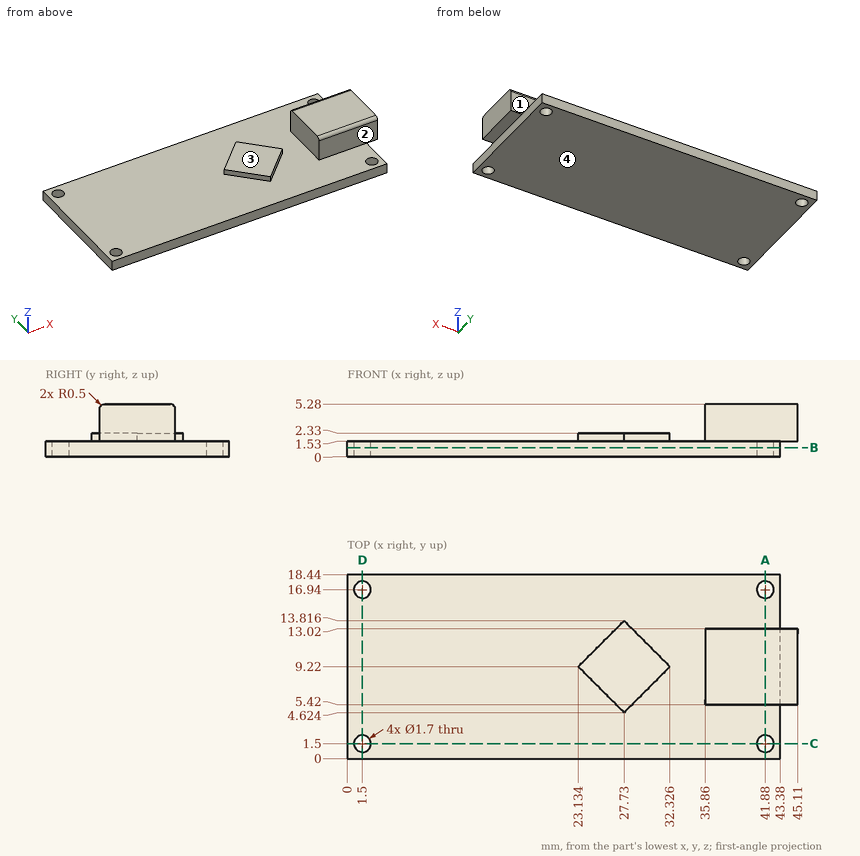
Source: three-view drawing plus pictorial views. Frame: mm from the lowest corner of the part. A direction names the side the tool comes from. Round coordinates to 2 decimals unless told otherwise and drop trailing zeros. Order: outer loops, then holes, each group sorted by start corner. A loop starts at its lowest first (then second) coordinate and runs counter-clockwise, first axis right, second up. Notation, with made-up numbers: (73, 2.25) - (106, 2.25) arc R24 cw to (106, 36.25) - close; hole circle Ø6 at (-29.75, -25). An arc over 180 degrees is marked (long way). Answer in a Markdown table with one row per item.
Item 1: Section query C-C (y = 1.5). Return the cut outline in (x, z).
Model answer:
| item | result |
|---|---|
| outline | (0, 0) - (0.65, 0) - (0.65, 1.53) - (0, 1.53) - close; (2.35, 0) - (41.03, 0) - (41.03, 1.53) - (2.35, 1.53) - close; (42.73, 0) - (43.38, 0) - (43.38, 1.53) - (42.73, 1.53) - close |
Item 2: Line query: line 1 (Y direction, x = 41.88, z = 1.2); line 2 (Z direction, x = 14, y = 13.75); line 3 (X direction, y = 16.5, z = 0.4). Output: solid intervals per line, ascending.
Model answer:
| item | result |
|---|---|
| line 1 | y = 0 to 0.65, 2.35 to 16.09, 17.79 to 18.44 |
| line 2 | z = 0 to 1.53 |
| line 3 | x = 0 to 0.77, 2.23 to 41.15, 42.61 to 43.38 |
Item 3: Section query A-A (x = 41.88). Return the cut outline in (y, z), then the cut area to 3 significant figures.
Model answer:
| item | result |
|---|---|
| outline | (0, 0) - (0.65, 0) - (0.65, 1.53) - (0, 1.53) - close; (2.35, 0) - (16.09, 0) - (16.09, 1.53) - (13.02, 1.53) - (13.02, 4.78) arc R0.5 ccw to (12.52, 5.28) - (5.92, 5.28) arc R0.5 ccw to (5.42, 4.78) - (5.42, 1.53) - (2.35, 1.53) - close; (17.79, 0) - (18.44, 0) - (18.44, 1.53) - (17.79, 1.53) - close |
| area | 51.4 mm² |
Item 4: Pin query (flat end, axial travel): pin 1 (5.5 mm diameter, centred on x = 13, y = 9.5, fed in from +Z); pin 2 (0.9 mm diameter, centred on x = 44.5, y = 7.5, fed in from -Z); pin 3 (7.5 mm diameter, centred on x = 29.5, y = 10.5, fed in from +Z); pin 4 (1.5 mm diameter, centred on x = 41.88, y = 16.94, fed in from -Z). Return the tip coordinate at first contact, or that it passes through.
Model answer:
| item | result |
|---|---|
| pin 1 | stops at z = 1.53 |
| pin 2 | stops at z = 1.53 |
| pin 3 | stops at z = 2.33 |
| pin 4 | passes through |
Item 5: Section query B-B (z = 0.9). Return the cut outline in (x, y).
Model answer:
| item | result |
|---|---|
| outline | (0, 0) - (43.38, 0) - (43.38, 18.44) - (0, 18.44) - close; hole circle Ø1.7 at (1.5, 1.5); hole circle Ø1.7 at (1.5, 16.94); hole circle Ø1.7 at (41.88, 1.5); hole circle Ø1.7 at (41.88, 16.94) |
Item 6: Reachability of the marked faces 1, 2, 3 and 4 from +Z, -Z, +X, -X, +Y, -Y: full face, straight path, thin tool, end or side. Return the list, or none.
Model answer:
| item | result |
|---|---|
| face 1 | +Z, +X, +Y |
| face 2 | +Z, +X, -Y |
| face 3 | +Z, -X, +Y, -Y |
| face 4 | -Z, +X, -X, +Y, -Y |
Item 7: Section query D-D (x = 1.5). Return the cut outline in (y, z), then the cut area to 3 significant figures.
Model answer:
| item | result |
|---|---|
| outline | (0, 0) - (0.65, 0) - (0.65, 1.53) - (0, 1.53) - close; (2.35, 0) - (16.09, 0) - (16.09, 1.53) - (2.35, 1.53) - close; (17.79, 0) - (18.44, 0) - (18.44, 1.53) - (17.79, 1.53) - close |
| area | 23.0 mm² |
